Geometry check sheet. Reference: the model listing, model coordinates, mm. Give positions to 0.01 mm unless a question says otherwise; leave off trailing zeros. Order: outer loops, then holes, each group sorted by start corner. A loop starts at its lowest first (then second) coordinate and runs counter-clockwise, first axis right, second up.
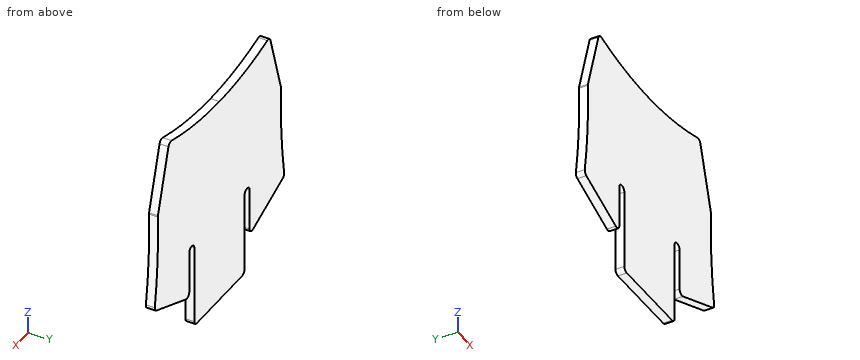
```python
from build123d import *

# Parameters (mm, degrees)
RESSALTO_EXTRUS_O1_DEPTH = 2


with BuildPart() as part:
    # Esboço1 → Ressalto-extrusão1 (new body)
    with BuildSketch(Plane(origin=(0, 0, 0), x_dir=(1, 0, 0), z_dir=(0, 1, 0))):
        with BuildLine():
            Line((9, 21.44797145), (-9, 21.44797145))
            ThreePointArc((-9, 21.44797145), (-9.707106781, 21.155078231), (-10, 20.44797145))
            Line((-10, 20.44797145), (-10, 2.4935203))
            ThreePointArc((-10, 2.4935203), (-11, 1.4935203), (-12, 2.4935203))
            Line((-12, 2.4935203), (-12, 11.963556295))
            ThreePointArc((-12, 11.963556295), (-12.441287452, 12.792917669), (-13.375680577, 12.890305508))
            Line((-13.375680577, 12.890305508), (-25.118348649, 8.130126323))
            ThreePointArc((-25.118348649, 8.130126323), (-25.611934385, 7.697721197), (-25.731213115, 7.052450978))
            ThreePointArc((-25.731213115, 7.052450978), (-24.623016259, -3.51887647), (-24.513147024, -14.147563739))
            ThreePointArc((-24.513147024, -14.147563739), (-24.505828612, -14.310453824), (-24.472135955, -14.469989225))
            Line((-24.472135955, -14.469989225), (-20.283702113, -28.518423408))
            ThreePointArc((-20.283702113, -28.518423408), (-19.807170843, -29.108999363), (-19.053198713, -29.194953058))
            ThreePointArc((-19.053198713, -29.194953058), (-9.617814606, -27.215907789), (0, -26.55202855))
            ThreePointArc((0, -26.55202855), (9.617814606, -27.215907789), (19.053198713, -29.194953058))
            ThreePointArc((19.053198713, -29.194953058), (19.807170843, -29.108999363), (20.283702113, -28.518423408))
            Line((20.283702113, -28.518423408), (24.472135955, -14.469989225))
            ThreePointArc((24.472135955, -14.469989225), (24.505828612, -14.310453824), (24.513147024, -14.147563739))
            ThreePointArc((24.513147024, -14.147563739), (24.623016259, -3.51887647), (25.731213115, 7.052450978))
            ThreePointArc((25.731213115, 7.052450978), (25.611934385, 7.697721197), (25.118348649, 8.130126323))
            Line((25.118348649, 8.130126323), (13.375680577, 12.890305508))
            ThreePointArc((13.375680577, 12.890305508), (12.441287452, 12.792917669), (12, 11.963556295))
            Line((12, 11.963556295), (12, 2.4935203))
            ThreePointArc((12, 2.4935203), (11, 1.4935203), (10, 2.4935203))
            Line((10, 2.4935203), (10, 20.44797145))
            ThreePointArc((10, 20.44797145), (9.707106781, 21.155078231), (9, 21.44797145))
        make_face()
    extrude(amount=RESSALTO_EXTRUS_O1_DEPTH)


solid = part.part
```
Q1. Thickness scan on L1, parallel to Z at x = -0.5, y = 1.7; L2, parallel to X at y = 0.9, z = 5.5; L3, parallel to Z at x = -18, y = 0.3. Record the ranges inside material, lowest first.
Q2. Cross-section at A-A, the plane y = 0.5. Record the boundary of the cut face in (x, z), and give its area (3 significant figures).
Q3. Gauge pin test, flat end, axial feed: P1, Ø0.6, axis at y = 1.5, z = -7.5, coming from the -X side. Record the tip position at first contact, or that the pin passes through.
Q4. Cross-section at C-C, the plane x = -14. Record the boundary of the cut face in (y, z).
Q5. Cross-section at B-B, the plane x = 11. Record the boundary of the cut face in (y, z).
Answers follow:
1. L1: z = -21.45 to 26.55
1. L2: x = -24.53 to 24.53
1. L3: z = -11.02 to 28.91
2. outline: (-25.73, -7.05) arc R1 ccw to (-25.12, -8.13) - (-13.38, -12.89) arc R1 ccw to (-12, -11.96) - (-12, -2.49) arc R1 cw to (-10, -2.49) - (-10, -20.45) arc R1 ccw to (-9, -21.45) - (9, -21.45) arc R1 ccw to (10, -20.45) - (10, -2.49) arc R1 cw to (12, -2.49) - (12, -11.96) arc R1 ccw to (13.38, -12.89) - (25.12, -8.13) arc R1 ccw to (25.73, -7.05) arc R112.98 cw to (24.51, 14.15) arc R1 ccw to (24.47, 14.47) - (20.28, 28.52) arc R1 ccw to (19.05, 29.19) arc R70 cw to (-19.05, 29.19) arc R1 ccw to (-20.28, 28.52) - (-24.47, 14.47) arc R1 ccw to (-24.51, 14.15) arc R112.98 cw to start
2. area: 2,020 mm2
3. P1: stops at x = -25.74
4. outline: (0, -12.64) - (2, -12.64) - (2, 27.97) - (0, 27.97) - close
5. outline: (0, -1.49) - (2, -1.49) - (2, 27.42) - (0, 27.42) - close
